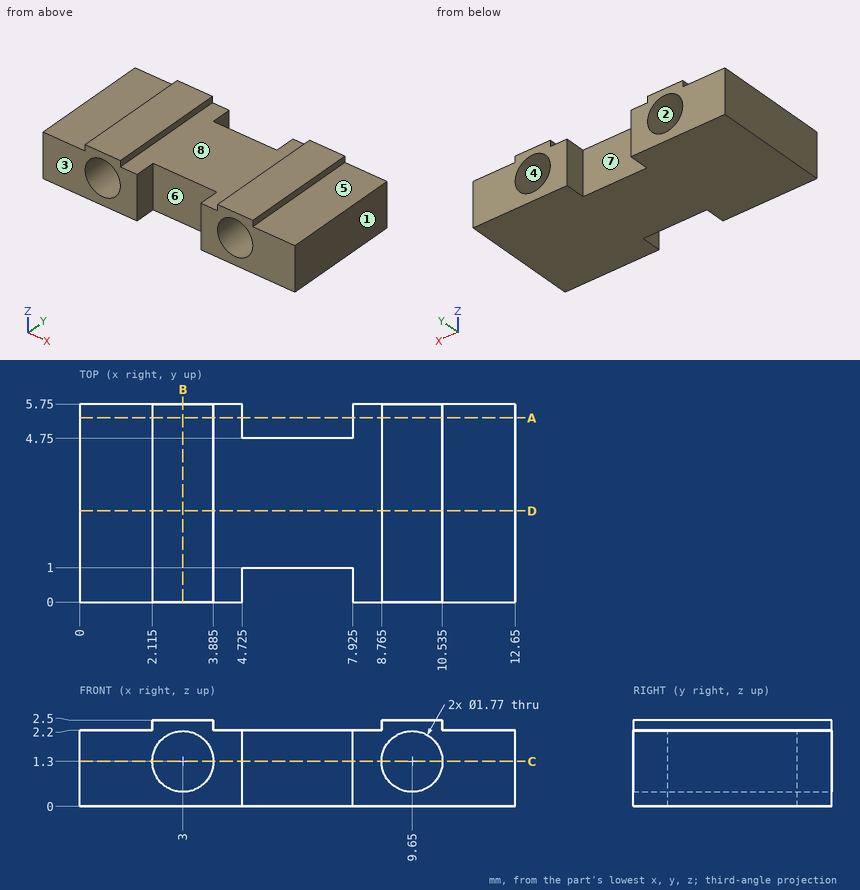
Source: three-view drawing plus pictorial views. Frame: mm from the lowest corner of the part. A direction names the side the tool comes from. Give positions to 0.01 mm unless a question says otherwise; leave off trailing zeros. Write each loop counter-clockwise with the first axis right and the second up, starting at its lowest first coordinate (ties: lowest second). Pieces come first, ordered by that corner, then holes.
(1) Access query for the marked faces 5, 6, 7 and 8. Directions: +Z, -Z, +X, -X, +Y, -Y. A direction counts if a zero-diameter tool reaches every point of the face in a straight line with its end or side. Return the directions, or none.
(2) Cut plane A-A, the plane y = 5.35. Return loops of the section in (x, z) (3 decimals).
(3) Mould query, pull axis X, two halves, no side actions, for the marked faces 1, 2, 3 and 4. Classes: released by +X, released by -X, zero draft, split by the parting line, or undercut.
(4) Ray query, line 1 (X direction, y = 4.1, z = 1.85); line 2 (X direction, y = 4.1, z = 2.1); line 3 (Z direction, x = 9.65, y = 2.95) (3 decimals). Return the intervals inside material, ascending.
(5) Cut plane C-C, the plane z = 1.3. Return loops of the section in (x, y) (3 decimals).
(6) First-contact query: P1, Ø1.1, axis at x = 12, y = 3.5, coming from the +Z side. Flat tip, straight axial feed; report the tip coordinate or a pass-through.
(7) Cut plane D-D, the plane y = 2.65. Return loops of the section in (x, z) (3 decimals), then the cut area to 3 significant figures.
(8) Cut plane B-B, the plane x = 3. Return loops of the section in (y, z) (3 decimals).
Values follow:
1. face 5: +Z, +X, +Y, -Y
1. face 6: +Z, -Z, -Y
1. face 7: +Z, -Z, +Y
1. face 8: +Z, +Y, -Y
2. outline: (0, 0) - (4.725, 0) - (4.725, 2.2) - (3.885, 2.2) - (3.885, 2.5) - (2.115, 2.5) - (2.115, 2.2) - (0, 2.2) - close; (7.925, 0) - (12.65, 0) - (12.65, 2.2) - (10.535, 2.2) - (10.535, 2.5) - (8.765, 2.5) - (8.765, 2.2) - (7.925, 2.2) - close; hole circle Ø1.77 at (3, 1.3); hole circle Ø1.77 at (9.65, 1.3)
3. face 1: released by +X
3. face 2: undercut
3. face 3: zero draft
3. face 4: undercut
4. line 1: x = 0 to 2.31, 3.69 to 8.96, 10.34 to 12.65
4. line 2: x = 0 to 2.62, 3.38 to 9.27, 10.03 to 12.65
4. line 3: z = 0 to 0.415, 2.185 to 2.5
5. outline: (0, 0) - (2.115, 0) - (2.115, 5.75) - (0, 5.75) - close; (3.885, 0) - (4.725, 0) - (4.725, 1) - (7.925, 1) - (7.925, 0) - (8.765, 0) - (8.765, 5.75) - (7.925, 5.75) - (7.925, 4.75) - (4.725, 4.75) - (4.725, 5.75) - (3.885, 5.75) - close; (10.535, 0) - (12.65, 0) - (12.65, 5.75) - (10.535, 5.75) - close
6. P1: stops at z = 2.2
7. outline: (0, 0) - (12.65, 0) - (12.65, 2.2) - (10.535, 2.2) - (10.535, 2.5) - (8.765, 2.5) - (8.765, 2.2) - (3.885, 2.2) - (3.885, 2.5) - (2.115, 2.5) - (2.115, 2.2) - (0, 2.2) - close; hole circle Ø1.77 at (3, 1.3); hole circle Ø1.77 at (9.65, 1.3)
7. area: 24.0 mm2
8. outline: (0, 0) - (5.75, 0) - (5.75, 0.415) - (0, 0.415) - close; (0, 2.185) - (5.75, 2.185) - (5.75, 2.5) - (0, 2.5) - close
